Geometry check sheet. Reference: the model listing, model coordinates, mm. A direction names the side the tool comes from. Give positions to 0.01 mm unless a question says otherwise; leave off trailing zeros. Loops run counter-clockwise (first coordinate to the right, second up) from the corner with the lowest first, then second, coordinate; pieces in that order, holes last. Notation, with made-up numbers: (-32, 1.5) - (-26, 1.5) arc R4 cw to (-26, 8.5) - close; hole circle Ø11 at (57.25, -37). An arc over 180 degrees is marked (long way). One line per question, with ' | ' between items. Start each with the question number.
from build123d import *

# Parameters (mm, degrees)
BOSS_EXTRUDE1_DEPTH = 25.4
SKETCH2_R           = 2.25
CUT_EXTRUDE1_DEPTH  = 6


with BuildPart() as part:
    # Sketch1 → Boss-Extrude1 (new body)
    with BuildSketch(Plane(origin=(0, 0, 0), x_dir=(1, 0, 0), z_dir=(0, 1, 0))):
        Polygon((-6.5, 18.750739811), (-1.5, 21.642901866), (-1.5, 32.503507515), (-6.5, 32.503507515), align=None)
        with BuildLine():
            Line((-1.5, -21.625070485), (-1.5, -14.221111068))
            ThreePointArc((-1.5, -14.221111068), (-14.3, 0), (-1.5, 14.221111068))
            Line((-1.5, 14.221111068), (-1.5, 21.642901866))
            Line((-1.5, 21.642901866), (-6.5, 18.750739811))
            Line((-6.5, 18.750739811), (-19.494691465, 11.234189098))
            Line((-19.494691465, 11.234189098), (-19.476438882, -11.265803499))
            Line((-19.476438882, -11.265803499), (-6.5, -18.743724782))
            Line((-6.5, -18.743724782), (-1.5, -21.625070485))
        make_face()
        Polygon((-1.5, -32.496492485), (-1.5, -21.625070485), (-6.5, -18.743724782), (-6.5, -32.496492485), align=None)
    extrude(amount=BOSS_EXTRUDE1_DEPTH)

    # Sketch2 → Cut-Extrude1 (cut, through all)
    with BuildSketch(Plane.ZY.offset(6.5)):
        with Locations((25.620108634, 18.7)):
            Circle(SKETCH2_R)
        with Locations((25.620108634, 6.7)):
            Circle(SKETCH2_R)
    cut_extrude1 = extrude(amount=-CUT_EXTRUDE1_DEPTH, mode=Mode.SUBTRACT)

    # Mirror1: Cut-Extrude1 across plane
    add(cut_extrude1.mirror(Plane.XY), mode=Mode.SUBTRACT)


solid = part.part
(1) Section check A-A, the plane y = 6.7. Record the boundary of the cut face in (x, z).
(2) Tool access check on faces 1 (the face through (-4.035, 5.331, -23.835)), 2 (the face through (-6.5, 13, -26)). Record the directions out of +Z, -Z, +X, -X, +Y, -Y that give a thin tool (end or side, any length) a straight path to the whole face; none if there is none.
(3) Depth check by flat-ended pin: pin 1 Ø1.5 at (y, z) = (21.5, -13) entering from -X; pin 2 Ø4 at (y, z) = (12, 25) entering from -X; pin 3 Ø6 at (y, z) = (10.5, -8.5) entering from +X; pin 4 Ø6 at (y, z) = (18.7, -25.62) entering from +X. Enter the tip coordinate at first touch or a pass-through.
(4) Section check D-D, the plane z = 25. Record the boundary of the cut face in (x, y).
(5) Mould release check, pull along Z, two halves, no side actions. Record for faces 3 (the face through (-4.035, 5.331, 23.835)), 4 (the face through (-12.906, 12.522, -15.045)), 5 (the face through (-6.5, 13, 26)): pulls with the +Z half, pulls with the -Z half, needs draft (parallel to the pull), parting line crosses it, or undercut.
(6) Material ranges on line 1 (Z direction, x = -6, y = 20.25); line 2 (Z direction, x = -4, y = 5); line 3 (X direction, y = 19.25, z = -22.5), recorded low to high.
(7) Section check C-C, the plane y = 14.5. Record the boundary of the cut face in (x, z).
(8) Section check B-B, the plane x = -4. Record the boundary of the cut face in (y, z).
Numbers:
1) outline: (-19.49, -11.23) - (-6.5, -18.75) - (-6.5, -23.37) - (-1.5, -23.37) - (-1.5, -14.22) arc R14.3 cw to (-1.5, 14.22) - (-1.5, 23.37) - (-6.5, 23.37) - (-6.5, 18.74) - (-19.48, 11.27) - close; (-6.5, -32.5) - (-1.5, -32.5) - (-1.5, -27.87) - (-6.5, -27.87) - close; (-6.5, 27.87) - (-1.5, 27.87) - (-1.5, 32.5) - (-6.5, 32.5) - close
2) face 1: +X, -X | face 2: -Z, -X, +Y, -Y
3) pin 1: x = -17.74 | pin 2: x = -6.5 | pin 3: x = -8.5 | pin 4: x = -1.5
4) outline: (-6.5, 0) - (-1.5, 0) - (-1.5, 4.54) - (-6.5, 4.54) - close; (-6.5, 8.86) - (-1.5, 8.86) - (-1.5, 16.54) - (-6.5, 16.54) - close; (-6.5, 20.86) - (-1.5, 20.86) - (-1.5, 25.4) - (-6.5, 25.4) - close
5) face 3: undercut | face 4: pulls with the -Z half | face 5: needs draft
6) line 1: -32.5 to -27.25, -23.99 to -12.98, 12.98 to 23.99, 27.25 to 32.5 | line 2: -32.5 to -27.09, -24.15 to -13.73, 13.73 to 24.15, 27.09 to 32.5 | line 3: -6.5 to -1.5
7) outline: (-19.49, -11.23) - (-6.5, -18.75) - (-6.5, -32.5) - (-1.5, -32.5) - (-1.5, -14.22) arc R14.3 cw to (-1.5, 14.22) - (-1.5, 32.5) - (-6.5, 32.5) - (-6.5, 18.74) - (-19.48, 11.27) - close
8) outline: (0, -32.5) - (25.4, -32.5) - (25.4, -13.73) - (0, -13.73) - close; (0, 13.73) - (25.4, 13.73) - (25.4, 32.5) - (0, 32.5) - close; hole circle Ø4.5 at (6.7, -25.62); hole circle Ø4.5 at (6.7, 25.62); hole circle Ø4.5 at (18.7, -25.62); hole circle Ø4.5 at (18.7, 25.62)
